Could you check a few things on this model? Use its own coordinates, in mm. A direction names the side the tool comes from. Give positions to 0.01 mm unless a question says otherwise; leave off trailing zeros. Order: outer loops, then holes, each group sorted by start corner. A loop starts at its lowest first (then second) coordinate and runs counter-clockwise, first axis right, second up. Notation, with made-up numbers: (-17.5, 27) -> (-0.5, 27) arc R35 cw to (-0.5, 60) -> close; hole circle Ø1 at (-24.75, 34). An arc over 180 degrees is marked (long way). Write each question's results on one line, items separated by ' | '.
```python
from build123d import *

# Parameters (mm, degrees)
SKETCH1_W           = 21.5
SKETCH1_H           = 44
BOSS_EXTRUDE1_DEPTH = 3
SKETCH1_3_W         = 10
SKETCH1_3_H         = 20
BOSS_EXTRUDE2_DEPTH = 1.5
BOSS_EXTRUDE3_DEPTH = 45.25
SKETCH2_W           = 10
SKETCH2_H           = 10
BOSS_EXTRUDE4_DEPTH = 3
CHAMFER1_SIZE       = 5.25


with BuildPart() as part:
    # Sketch1 → Boss-Extrude1 (new body)
    with BuildSketch(Plane(origin=(0, 0, 0), x_dir=(1, 0, 0), z_dir=(0, 1, 0))):
        with Locations((-10.75, 22)):
            Rectangle(SKETCH1_W, SKETCH1_H)
    extrude(amount=BOSS_EXTRUDE1_DEPTH)

    # Sketch1<3> → Boss-Extrude2 (add)
    with BuildSketch(Plane(origin=(0, 0, 0), x_dir=(1, 0, 0), z_dir=(0, 1, 0))):
        with Locations((5, 22)):
            Rectangle(SKETCH1_3_W, SKETCH1_3_H)
    extrude(amount=BOSS_EXTRUDE2_DEPTH)

    # Sketch1<4> → Boss-Extrude3 (add)
    with BuildSketch(Plane(origin=(0, 0, 0), x_dir=(1, 0, 0), z_dir=(0, 1, 0))):
        Polygon((-14.5, -3), (-14.5, 0), (-21.5, 0), (-21.5, 7), (-24.5, 7), (-24.5, -3), align=None)
        Polygon((-24.5, 37), (-21.5, 37), (-21.5, 44), (-14.5, 44), (-14.5, 47), (-24.5, 47), align=None)
    extrude(amount=BOSS_EXTRUDE3_DEPTH)

    # Sketch2 → Boss-Extrude4 (add)
    with BuildSketch(Plane(origin=(0, 45.25, 0), x_dir=(1, 0, 0), z_dir=(0, 1, 0))):
        with Locations((-19.5, 2)):
            Rectangle(SKETCH2_W, SKETCH2_H)
        with Locations((-19.5, 42)):
            Rectangle(SKETCH2_W, SKETCH2_H)
    extrude(amount=BOSS_EXTRUDE4_DEPTH)

    # Chamfer1
    chamfer1_edges = [part.edges().sort_by_distance(p)[0] for p in [
        (-21.5, 24.125, 0),
        (-21.5, 24.125, -44),
    ]]
    chamfer(chamfer1_edges, length=CHAMFER1_SIZE)


solid = part.part
```
Q1. I'm going to push flat-ended pins straight in: pin 1 Ø0.5 at (y, z) = (16, -38) entering from +X; pin 2 Ø8 at (y, z) = (22.5, -41) entering from +X; pin 3 Ø2.5 at (y, z) = (2, -24) entering from -X. Where does each tip first touch, or does it pass through?
Here are the results:
pin 1: stops at x = -21.5 | pin 2: stops at x = -14.5 | pin 3: stops at x = -21.5
Q2. I need wall thicknesses on line 1 along Z through (x, y) = (-15, 15.5); line 2 along Y through (x, z) = (-19.5, -4.5); line 3 along X through (y, z) = (14, 1). Which ranges of each line are inside material? Lowest first, please.
Here are the results:
line 1: z = -47 to -44, 0 to 3 | line 2: y = 0 to 3, 45.25 to 48.25 | line 3: x = -24.5 to -14.5
Q3. Thinking about a two-plate mould opening in Y: for faces 1 (the flat face through (-7, 1, 0)), 2 (the flat face through (-18.91, 23.83, -41.34)), 3 (the flat face through (-11, 0, -22)), which applies, +Y half, -Y half, draft (parallel to the pull), parting line (faces both ways), or undercut?
Here are the results:
face 1: draft | face 2: undercut | face 3: -Y half
Q4. Suppose I cut it at A-A on y = 15.5. Please give me the cut outline in (x, z), and give its area (3 significant figures).
Here are the results:
outline: (-24.5, -47) -> (-14.5, -47) -> (-14.5, -44) -> (-16.25, -44) -> (-21.5, -38.75) -> (-21.5, -37) -> (-24.5, -37) -> close; (-24.5, -7) -> (-21.5, -7) -> (-21.5, -5.25) -> (-16.25, 0) -> (-14.5, 0) -> (-14.5, 3) -> (-24.5, 3) -> close | area: 130 mm²
Q5. For faces 4 (the flat face through (5, 1, -12)), 5 (the flat face through (5, 1, -32)), 6 (the flat face through (-18.84, 23.83, -2.59)), 7 (the flat face through (5, 1.5, -22)), which set-ups out of +Z, -Z, +X, -X, +Y, -Y let a thin tool reach every point of the face, with its end or its side?
Here are the results:
face 4: +Z, +X, +Y, -Y | face 5: -Z, +X, +Y, -Y | face 6: +X | face 7: +Z, -Z, +X, +Y
Q6. Suppose I cut it at C-C on x = -17.5. Please give me the cut outline in (y, z), and give its area (3 significant figures).
Here are the results:
outline: (0, -47) -> (48.25, -47) -> (48.25, -37) -> (45.25, -37) -> (45.25, -42.75) -> (3, -42.75) -> (3, -1.25) -> (45.25, -1.25) -> (45.25, -7) -> (48.25, -7) -> (48.25, 3) -> (0, 3) -> close | area: 569 mm²
Q7. Suppose I cut it at B-B on z = -40.5. Please give me the cut outline in (x, y).
Here are the results:
outline: (-24.5, 0) -> (0, 0) -> (0, 3) -> (-19.75, 3) -> (-19.75, 45.25) -> (-14.5, 45.25) -> (-14.5, 48.25) -> (-24.5, 48.25) -> close
Q8. Suppose I cut it at D-D on z = -4. Please give me the cut outline in (x, y).
Here are the results:
outline: (-24.5, 0) -> (0, 0) -> (0, 3) -> (-20.25, 3) -> (-20.25, 45.25) -> (-14.5, 45.25) -> (-14.5, 48.25) -> (-24.5, 48.25) -> close
